Verification items for the finished model (mm, model axes). A direction names the side the tool comes from. Round coordinates to 2 decimals unless told otherwise and drop trailing zeros. Order: outer loops, then holes, each group sorted by start corner. A loop starts at its lowest first (then second) coordinate and runs counter-clockwise, first axis right, second up. Notation, with made-up numbers: (35, 55.25) -> (51, 55.25) arc R13 cw to (51, 67.25) -> close; hole circle Ø7 at (17, 77). An arc over 180 degrees is marked (long way). Put each result on its own line as item: value.
Autodesk Inventor part; units mm, degrees
ref_plane "YZ Plane" through (0, 0, 0) normal (1, 0, 0) x (0, 1, 0)
ref_plane "XZ Plane" through (0, 0, 0) normal (0, 1, 0) x (-1, 0, 0)
ref_plane "XY Plane" through (0, 0, 0) normal (0, 0, 1) x (1, 0, 0)
sketch "Sketch1" plane through (0, 0, 0) normal (0, 0, 1) x (1, 0, 0)
  line L0 (-2.0384, 1.8879) -> (2.0592, 1.8879)
  line L1 (2.0592, 1.8879) -> (2.0592, -1.9739)
  line L2 (2.0592, -1.9739) -> (-2.0384, -1.9739)
  line L3 (-2.0384, -1.9739) -> (-2.0384, 1.8879)
  arc A0 (2.0592, -1.9739) -> (2.0592, 1.8879) centre (-0.1442, -0.043) ccw
  arc A1 (-2.0384, 1.8879) -> (-2.0384, -1.9739) centre (-0.6409, -0.043) ccw
  line L4 (6, 11.5957) -> (-6.1442, 11.5957)
  line L5 (-6.1442, 11.5957) -> (-6.1442, -176.351)
  line L6 (-6.1442, -176.351) -> (6, -176.351)
  line L7 (6, -176.351) -> (6, 11.5957)
  point P0 (0, 0)
  dimension "d2" = 6
  dimension "d3" = 6
extrude "Extrusion1" add sketch "Sketch1" along normal blind 10
sketch "Sketch2" plane through (-6.1442, -176.351, 0) normal (-1, 0, 0) x (0, 0, 1)
  line L0 (3.5426, 125.3505) -> (1.5426, 125.3505)
  line L1 (1.5426, 125.3505) -> (1.5426, 120.3505)
  line L2 (1.5426, 120.3505) -> (3.5426, 120.3505)
  line L3 (3.5426, 120.3505) -> (3.5426, 125.3505)
  line L4 (3.5426, 70.3505) -> (1.5426, 70.3505)
  line L5 (1.5426, 70.3505) -> (1.5426, 65.3505)
  line L6 (1.5426, 65.3505) -> (3.5426, 65.3505)
  line L7 (3.5426, 65.3505) -> (3.5426, 70.3505)
  circle A0 centre (4.5547, 34.075) radius 2.5
  circle A1 centre (4.5547, 12.3917) radius 2.5
  point P0 (0, 176.351)
  dimension "d4" = 2
  dimension "d5" = 5
  dimension "d6" = 2
  dimension "d7" = 5
  dimension "d10" = 50
  dimension "d11" = 5
  dimension "d12" = 5
extrude "Extrusion2" cut sketch "Sketch2" against normal through all
sketch "Sketch3" plane through (-6.1442, -176.351, 0) normal (-1, 0, 0) x (0, 0, 1)
  point P0 (0, 176.351)
sketch "Sketch4" plane through (0, 0, 0) normal (0, 0, -1) x (-1, 0, 0)
  circle A0 centre (0, 0) radius 4.5
  dimension "d13" = 9
extrude "Extrusion3" add sketch "Sketch4" along normal blind 5.2375 and the other way blind 10
sketch "Sketch5" plane through (0, 0, 0) normal (0, 0, -1) x (-1, 0, 0)
  line L0 (2.0992, 1.8119) -> (-1.885, 1.8119)
  line L1 (-1.885, 1.8119) -> (-1.885, -1.9325)
  line L2 (-1.885, -1.9325) -> (2.0992, -1.9325)
  line L3 (2.0992, -1.9325) -> (2.0992, 1.8119)
  arc A0 (2.0992, -1.9325) -> (2.0992, 1.8119) centre (0.2308, -0.0603) ccw
  arc A1 (-1.885, 1.8119) -> (-1.885, -1.9325) centre (-0.0175, -0.0603) ccw
  point P0 (0, 0)
extrude "Extrusion4" cut sketch "Sketch5" along normal blind 5.2375 and the other way blind 4.2065
fillet "Fillet1" radius 2 4 edges at (6, 11.5957, 5) (-6.1442, 11.5957, 5) (-6.1442, -176.351, 5) (6, -176.351, 5)
properties part number "Arm"
Item 1: Sectioned sample at C-C, the plane y = -158. Record the boundary of the cut face in (x, z).
Geometry check:
outline: (-6.14, 0) -> (6, 0) -> (6, 10) -> (-6.14, 10) -> close
Item 2: Sectioned sample at A-A, the plane x = 0. Record the boundary of the cut face in (y, z).
Geometry check:
outline: (-176.35, 0) -> (-4.5, 0) -> (-4.5, -5.24) -> (-1.93, -5.24) -> (-1.93, 4.21) -> (1.81, 4.21) -> (1.81, -5.24) -> (4.5, -5.24) -> (4.5, 0) -> (11.6, 0) -> (11.6, 10) -> (-176.35, 10) -> close; hole circle Ø5 at (-163.96, 4.55); hole circle Ø5 at (-142.28, 4.55); hole (-111, 1.54) -> (-106, 1.54) -> (-106, 3.54) -> (-111, 3.54) -> close; hole (-56, 1.54) -> (-51, 1.54) -> (-51, 3.54) -> (-56, 3.54) -> close
Item 3: Tool access check on faces 1 (the face through (-2.876, -0.031, -0.449)), 2 (the face through (6, -84, 5)), 3 (the face through (0, -109, 3.543)). Record the directions out of +Z, -Z, +X, -X, +Y, -Y that give a thin tool (end or side, any length) a straight path to the whole face; none if there is none.
Geometry check:
face 1: -Z
face 2: +Z, -Z, +X, +Y, -Y
face 3: +X, -X
Item 4: Sectioned sample at B-B, the plane y = 0. Record the boundary of the cut face in (x, z), then the cut area to 3 significant figures.
Geometry check:
outline: (-6.14, 0) -> (-4.5, 0) -> (-4.5, -5.24) -> (-2.88, -5.24) -> (-2.88, 4.21) -> (2.66, 4.21) -> (2.66, -5.24) -> (4.5, -5.24) -> (4.5, 0) -> (6, 0) -> (6, 10) -> (-6.14, 10) -> close
area: 116 mm2
Item 5: Release check for a two-part mould opening along Y. For faces 4 (the face through (0, 2, -5.238)), 5 (the face through (0.59, -4.46, -2.58)), 6 (the face through (0, 1.812, 0)) record: pulls with the +Y half, pulls with the -Y half, needs draft (parallel to the pull), parting line crosses it, or undercut.
Geometry check:
face 4: needs draft
face 5: parting line crosses it
face 6: undercut
Item 6: Material ranges on line 1 along Z through (x, y) = (-1.25, -109); line 2 along Y through (x, z) = (1.25, 1); line 3 along Y through (x, z) = (2.5, 5.5), recorded low to high.
Geometry check:
line 1: 0 to 1.54, 3.54 to 10
line 2: -176.35 to -1.93, 1.81 to 11.6
line 3: -176.35 to -166.27, -161.64 to -144.59, -139.96 to 11.6
Item 7: Depth check by flat-ended pin: pin 1 Ø4 at (x, y) = (-2.5, -53) entering from -Z; pin 2 Ø3 at (x, y) = (0, -0.5) entering from -Z. Enter the tip coordinate at first touch or a pass-through.
Geometry check:
pin 1: z = 0
pin 2: z = -5.24
